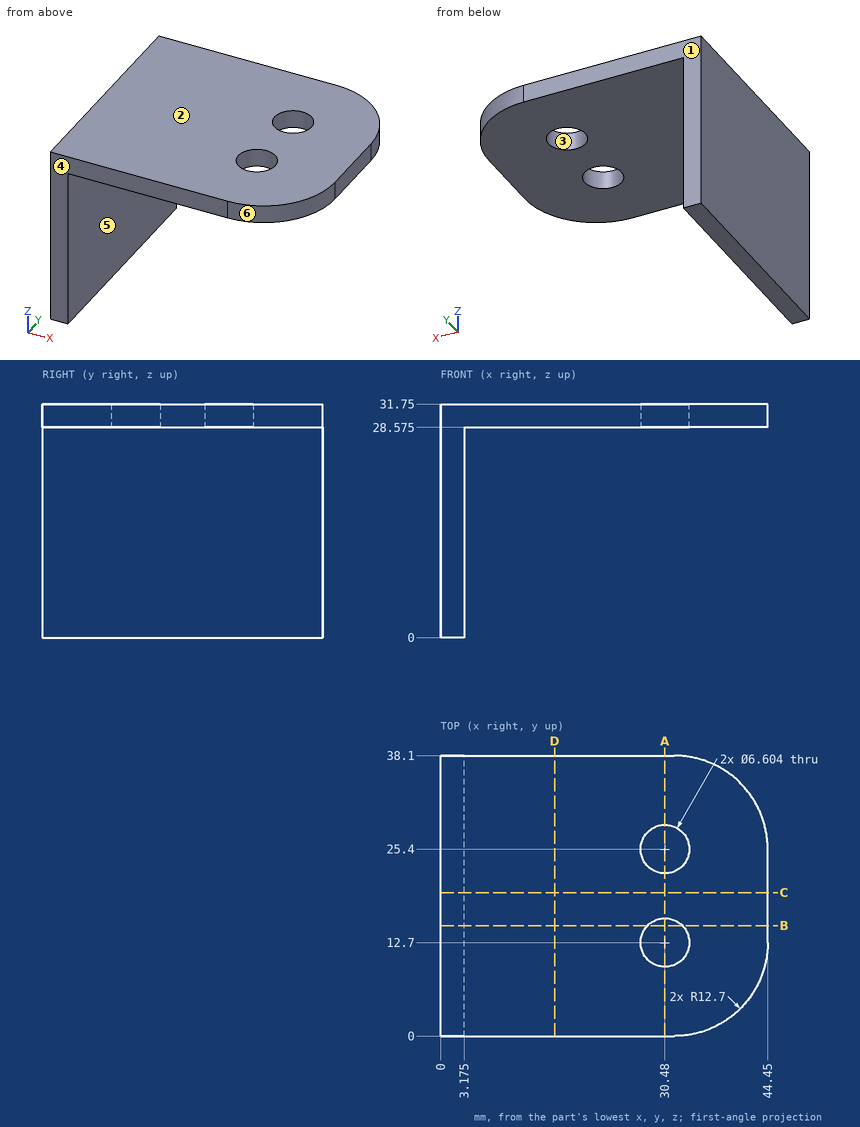
Verification items for this drawing (mm, ordinates from the low corner). A direction names the side the tool comes from. Give positions to 0.01 mm unless a question says otherwise; leave off trailing zeros. Loops run counter-clockwise (first coordinate to the right, second up) from the corner with the lowest first, then second, coordinate; pieces in that order, holes last. Notation, with made-up numbers: M -13,51.25 L -5,51.25 A18 ccw -5,68.25 Z; hole C 65.25,58 d5. An arc over 180 degrees is marked long. Write item = value, one per line.
(1) Gauge pin test, flat ends, axial feed: pin 1 Ø8.5 at (y, z) = (26.5, 16.5) entering from +X (3 decimals); pin 2 Ø10 at (x, y) = (30.5, 10) entering from -Z (3 decimals); pin 3 Ø5 at (x, z) = (37, 28.5) entering from -Y; pin 4 Ø5.5 at (x, y) = (30.48, 25.4) entering from +Z. Record the tip position at first contact, or that the pin passes through.
Answer below:
pin_1 = 3.175
pin_2 = 28.575
pin_3 = 0.3
pin_4 = through
(2) Tool access check on the marked faces 5 and 6. Record the directions out of +Z, -Z, +X, -X, +Y, -Y that give a thin tool (end or side, any length) a straight path to the whole face; none if there is none.
Answer below:
face_5 = -Z, +X, +Y, -Y
face_6 = +Z, -Z, +X, -Y
(3) Release check for a two-part mould opening along Y. For the marked faces 1, 2, 3 and 4 record: released by +Y, released by -Y, zero draft, split by the parting line, or undercut.
Answer below:
face_1 = released by +Y
face_2 = zero draft
face_3 = undercut
face_4 = released by -Y
(4) Sectioned sample at B-B, the plane y = 15. Record the cut outline in (x, z) (3 decimals), plus the area to 3 significant figures.
Answer below:
outline = M 0,0 L 3.175,0 L 3.175,28.575 L 28.111,28.575 L 28.111,31.75 L 0,31.75 Z; M 32.849,28.575 L 44.45,28.575 L 44.45,31.75 L 32.849,31.75 Z
area = 217 mm2
(5) Sectioned sample at A-A, the plane x = 30.48. Record the cut outline in (y, z) (3 decimals).
Answer below:
outline = M 0,28.575 L 9.398,28.575 L 9.398,31.75 L 0,31.75 Z; M 16.002,28.575 L 22.098,28.575 L 22.098,31.75 L 16.002,31.75 Z; M 28.702,28.575 L 38.1,28.575 L 38.1,31.75 L 28.702,31.75 Z
(6) Sectioned sample at C-C, the plane y = 19.5. Record the cut outline in (x, z) (3 decimals).
Answer below:
outline = M 0,0 L 3.175,0 L 3.175,28.575 L 44.45,28.575 L 44.45,31.75 L 0,31.75 Z
(7) Sectioned sample at D-D, the plane x = 15.5. Record the cut outline in (y, z) (3 decimals).
Answer below:
outline = M 0,28.575 L 38.1,28.575 L 38.1,31.75 L 0,31.75 Z
(8) Material ranges on line 1 (Y direction, x = 30.48, z = 31.05); line 2 (Z direction, x = 22.5, y = 7) (3 decimals), recorded low to high. Write a range as [from, to].
Answer below:
line_1 = [0, 9.4], [16, 22.1], [28.7, 38.1]
line_2 = [28.575, 31.75]
